```python
from build123d import *

# Parameters (mm, degrees)
SKETCH1_W           = 94
SKETCH1_H           = 57
BOSS_EXTRUDE1_DEPTH = 1
BOSS_EXTRUDE3_DEPTH = 30
SKETCH5_W           = 0.7
SKETCH5_H           = 1
BOSS_EXTRUDE4_DEPTH = 92
SKETCH6_W           = 46
SKETCH6_H           = 11
CUT_EXTRUDE2_DEPTH  = 30
SKETCH7_W           = 10
SKETCH7_H           = 2
BOSS_EXTRUDE5_DEPTH = 2
SKETCH8_W           = 25
SKETCH8_H           = 13
CUT_EXTRUDE3_DEPTH  = 2
SKETCH9_W           = 38
SKETCH9_H           = 1
BOSS_EXTRUDE6_DEPTH = 1
SKETCH10_W          = 1
SKETCH10_H          = 1
BOSS_EXTRUDE7_DEPTH = 50
BOSS_EXTRUDE8_DEPTH = 1
SKETCH13_W          = 94
SKETCH13_H          = 57
BOSS_EXTRUDE9_DEPTH = 1


with BuildPart() as part:
    # Sketch1 → Boss-Extrude1 (new body)
    with BuildSketch(Plane(origin=(0, 0, 0), x_dir=(1, 0, 0), z_dir=(0, 1, 0))):
        with Locations((-9.450515464, -3.911340206)):
            Rectangle(SKETCH1_W, SKETCH1_H)
    extrude(amount=BOSS_EXTRUDE1_DEPTH)

    # Sketch2 → Boss-Extrude3 (add)
    with BuildSketch(Plane(origin=(0, 1, 0), x_dir=(1, 0, 0), z_dir=(0, 1, 0))):
        Polygon((-56.450515464, 24.588659794), (37.549484536, 24.588659794), (37.549484536, -32.411340206), (-56.450515464, -32.411340206), (-56.450515464, -30.411340206), (-54.450515464, -30.411340206), (35.549484536, -30.411340206), (35.549484536, 22.588659794), (-54.450515464, 22.588659794), (-56.450515464, 22.588659794), align=None)
    extrude(amount=BOSS_EXTRUDE3_DEPTH)

    # Sketch5 → Boss-Extrude4 (add)
    with BuildSketch(Plane.ZY.offset(56.450515464)):
        with Locations((-22.238659794, 5.5)):
            Rectangle(SKETCH5_W, SKETCH5_H)
        with Locations((30.061340206, 5.5)):
            Rectangle(SKETCH5_W, SKETCH5_H)
    extrude(amount=-BOSS_EXTRUDE4_DEPTH)

    # Sketch6 → Cut-Extrude2 (cut)
    with BuildSketch(Plane(origin=(0, 0, -24.588659794), x_dir=(-1, 0, 0), z_dir=(0, 0, -1))):
        with Locations((-7.549484536, 20.5)):
            Rectangle(SKETCH6_W, SKETCH6_H)
    extrude(amount=-CUT_EXTRUDE2_DEPTH, mode=Mode.SUBTRACT)

    # Sketch7 → Boss-Extrude5 (add)
    with BuildSketch(Plane(origin=(0, 31, 0), x_dir=(1, 0, 0), z_dir=(0, 1, 0))):
        with Locations((-51.450515464, 23.588659794)):
            Rectangle(SKETCH7_W, SKETCH7_H)
        with Locations((-23.450515464, 23.588659794)):
            Rectangle(SKETCH7_W, SKETCH7_H)
        with Locations((4.549484536, 23.588659794)):
            Rectangle(SKETCH7_W, SKETCH7_H)
        with Locations((32.549484536, 23.588659794)):
            Rectangle(SKETCH7_W, SKETCH7_H)
        with Locations((-51.450515464, -31.411340206)):
            Rectangle(SKETCH7_W, SKETCH7_H)
        with Locations((-23.450515464, -31.411340206)):
            Rectangle(SKETCH7_W, SKETCH7_H)
        with Locations((4.549484536, -31.411340206)):
            Rectangle(SKETCH7_W, SKETCH7_H)
        with Locations((32.549484536, -31.411340206)):
            Rectangle(SKETCH7_W, SKETCH7_H)
    extrude(amount=BOSS_EXTRUDE5_DEPTH)

    # Sketch8 → Cut-Extrude3 (cut)
    with BuildSketch(Plane(origin=(37.549484536, 0, 0), x_dir=(0, 0, -1), z_dir=(1, 0, 0))):
        with Locations((-3.911340206, 15.5)):
            Rectangle(SKETCH8_W, SKETCH8_H)
    extrude(amount=-CUT_EXTRUDE3_DEPTH, mode=Mode.SUBTRACT)

    # Sketch9 → Boss-Extrude6 (add)
    with BuildSketch(Plane.ZY.offset(-35.549484536)):
        with Locations((11.411340206, 23.5)):
            Rectangle(SKETCH9_W, SKETCH9_H)
    extrude(amount=BOSS_EXTRUDE6_DEPTH)

    # Sketch10 → Boss-Extrude7 (add)
    with BuildSketch(Plane.ZY.offset(-34.549484536)):
        with Locations((29.911340206, 23.5)):
            Rectangle(SKETCH10_W, SKETCH10_H)
    extrude(amount=BOSS_EXTRUDE7_DEPTH)

    # Sketch11 → Boss-Extrude8 (add)
    with BuildSketch(Plane(origin=(0, 25.7, 0), x_dir=(1, 0, 0), z_dir=(0, 1, 0))):
        Polygon((34.549484536, 7.588659794), (35.549484536, 7.588659794), (35.549484536, -30.411340206), (-15.450515464, -30.411340206), (-15.450515464, -29.411340206), (34.549484536, -29.411340206), align=None)
    extrude(amount=BOSS_EXTRUDE8_DEPTH)

    # Sketch13 → Boss-Extrude9 (add)
    with BuildSketch(Plane.XZ):
        with Locations((-9.450515464, 3.911340206)):
            Rectangle(SKETCH13_W, SKETCH13_H)
    extrude(amount=BOSS_EXTRUDE9_DEPTH)


solid = part.part
```
Check sheet for the modelled part. Datum: model origin and axes. Units: mm. A direction names the side the tool comes from. Coordinates: 2 decimals unless noted, no trailing zeros. Loops run counter-clockwise (first coordinate to the right, second up) from the corner with the lowest first, then second, coordinate; pieces in that order, holes last. Notation, with made-up numbers: M 9,26.5 L 44,26.5 A16 ccw 44,31.5 Z; hole C -6.5,44.25 d1. An arc over 180 degrees is marked long. Answer as a JSON object with one key per item and string values.
1. Depth check by flat-ended pin: P1, Ø12, axis at x = -27, z = 4, coming from the +Y side; P2, Ø12, axis at y = 24.5, z = 5.5, coming from the -X side; P3, Ø2, axis at x = -34, z = 31.5, coming from the +Y side. Enter the tip coordinate at first touch or a pass-through.
Outcome:
{"P1": "y = 1", "P2": "x = 34.55", "P3": "y = 31"}
2. Scan lines: L1, parallel to Z at x = -43, y = 22; L2, parallel to Y at x = 12, z = 2; L3, parallel to X at y = 7, z = 0.5. Record each from-to range of solid material in increasing order. Write a range as from..to.
Outcome:
{"L1": "-24.59..-22.59, 30.41..32.41", "L2": "-1..1", "L3": "35.55..37.55"}
3. Sectioned sample at C-C on z = 13. Record the cut outline in (x, y), and give its area (3 significant figures).
Outcome:
{"outline": "M -56.45,-1 L 37.55,-1 L 37.55,9 L 35.55,9 L 35.55,1 L -56.45,1 Z; M 34.55,23 L 35.55,23 L 35.55,22 L 37.55,22 L 37.55,31 L 35.55,31 L 35.55,26.7 L 34.55,26.7 L 34.55,25.7 L 35.55,25.7 L 35.55,24 L 34.55,24 Z", "area": "224 mm²"}
4. Sectioned sample at D-D on y = 20. Record the cut outline in (x, z), and give its area (3 significant figures).
Outcome:
{"outline": "M -56.45,-24.59 L -15.45,-24.59 L -15.45,-22.59 L -56.45,-22.59 Z; M -56.45,30.41 L 35.55,30.41 L 35.55,16.41 L 37.55,16.41 L 37.55,32.41 L -56.45,32.41 Z; M 30.55,-24.59 L 37.55,-24.59 L 37.55,-8.59 L 35.55,-8.59 L 35.55,-22.59 L 30.55,-22.59 Z", "area": "340 mm²"}
5. Sectioned sample at B-B on y = 12.5. Record the cut outline in (x, z).
Outcome:
{"outline": "M -56.45,-24.59 L 37.55,-24.59 L 37.55,-8.59 L 35.55,-8.59 L 35.55,-22.59 L -56.45,-22.59 Z; M -56.45,30.41 L 35.55,30.41 L 35.55,16.41 L 37.55,16.41 L 37.55,32.41 L -56.45,32.41 Z"}
6. Release check for a two-part mould opening along Y. For faces 5 (the flat face through (9.549, 32, -24)), 6 (the flat face through (19, 31, 31)), 7 (the flat face through (22, 23, 30)) record: pulls with the +Y half, pulls with the -Y half, needs draft (parallel to the pull), parting line crosses it, or undercut.
Outcome:
{"face 5": "needs draft", "face 6": "pulls with the +Y half", "face 7": "undercut"}
7. Sectioned sample at A-A on x = 6. Record the cut outline in (y, z), and give its area (3 significant figures).
Outcome:
{"outline": "M -1,-24.59 L 15,-24.59 L 15,-22.59 L 6,-22.59 L 6,-21.89 L 5,-21.89 L 5,-22.59 L 1,-22.59 L 1,30.41 L 5,30.41 L 5,29.71 L 6,29.71 L 6,30.41 L 23,30.41 L 23,29.41 L 24,29.41 L 24,30.41 L 25.7,30.41 L 25.7,29.41 L 26.7,29.41 L 26.7,30.41 L 33,30.41 L 33,32.41 L -1,32.41 Z; M 26,-24.59 L 33,-24.59 L 33,-22.59 L 26,-22.59 Z", "area": "223 mm²"}
8. Access from +Z, -Z, +X, -X, +Y, -Y to the whole of each face (thin tool, end or side, straight path). Record for faces 1 (the flat face through (37, 9, 4)), 2 (the flat face through (19, 31, -24)), 3 (the flat face through (30.549, 20, -24)), 4 (the flat face through (22, 24, 30)).
Outcome:
{"face 1": "+X, -X", "face 2": "+Z, -Z, +Y", "face 3": "-Z", "face 4": "-X"}
